from build123d import *

# Parameters (mm, degrees)
SKETCH2_R           = 12.5
SKETCH2_R_2         = 10
BOSS_EXTRUDE3_DEPTH = 90
SKETCH3_R           = 12.5
BOSS_EXTRUDE4_DEPTH = 30
BOSS_EXTRUDE5_DEPTH = 75


with BuildPart() as part:
    # Sketch2 → Boss-Extrude3 (new body)
    with BuildSketch(Plane(origin=(0, 0, 0), x_dir=(1, 0, 0), z_dir=(0, 1, 0))):
        with Locations(Location((0, 0, 0), (0, 0, 90))):
            Circle(SKETCH2_R)
        with Locations(Location((0, 0, 0), (0, 0, 90))):
            Circle(SKETCH2_R_2, mode=Mode.SUBTRACT)
    extrude(amount=BOSS_EXTRUDE3_DEPTH)

    # Sketch3 → Boss-Extrude4 (add)
    with BuildSketch(Plane(origin=(0, 90, 0), x_dir=(1, 0, 0), z_dir=(0, 1, 0))):
        with Locations(Location((0, 0, 0), (0, 0, 90))):
            Circle(SKETCH3_R)
    extrude(amount=BOSS_EXTRUDE4_DEPTH)

    # Sketch5 → Boss-Extrude5 (add, symmetric)
    with BuildSketch(Plane.XY):
        Polygon((-1, 90), (1, 90), (1, 120), (0, 165), (-1, 120), align=None)
    extrude(amount=BOSS_EXTRUDE5_DEPTH, both=True)


solid = part.part
The model under review builds one solid part; all positions refer to its coordinate system, in mm. A direction names the side the tool comes from. Round coordinates to 2 decimals unless told otherwise and drop trailing zeros. Write each loop counter-clockwise with the first axis right and the second up, starting at its lowest first coordinate (ties: lowest second). Pieces come first, ordered by that corner, then holes. Notation, with made-up numbers: M 86.5,-34.5 L 104.5,-34.5 A12 ccw 104.5,-17.5 Z; hole C 39,-1 d10. An arc over 180 degrees is marked long. Answer as CSV lines item,"result". Start each with the question number.
Q1. Consider section B-B, the plane z = 0. Give the boundary of the cut face in (x, y), then the cut area to 4 significant figures.
Q2. The part is to be moulded in two halves that separate along X. For faces 5 (the face through (1, 105, -43)), 6 (the face through (9.76, 44.37, 2.17)), 7 (the face through (5, 120, 0)), say which applies: +X half, -X half, draft (parallel to the pull), parting line (faces both ways), or undercut.
Q3. Consider section A-A, the plane y = 19. Give the boundary of the cut face in (x, z), then the cut area to 3 significant figures.
Q4. Wall thickness on line 1 along X through (y, z) = (29.5, 0); line 2 along Z through (x, y) = (6.75, 40); line 3 along Z through (x, y) = (-5.75, 21): over which ranges is each line inside the solid? List them lowest first.
Q5. Consider section C-C, the plane x = 5. Give the boundary of the cut face in (y, z).
Q6. Clearance check with flat-ended pins moving along their axes: P1, Ø9, axis at y = 111.5, z = 52, coming from the +X side; P2, Ø1, axis at x = -9, y = 94.5, coming from the -Z side; P3, Ø0.6, axis at x = 0, z = 36.5, coming from the -Y side. State where each tip first meets the part, or that it passes through.
Q7. Tool access review of faces 1 (the face through (1, 105, 44)), 2 (the face through (-1, 105, -43)), 3 (the face through (0, 90, 0)), 4 (the face through (-1, 105, 44)): name each direction out of +Z, -Z, +X, -X, +Y, -Y from which nothing blocks a thin tool from reaching the whole face with its end or side.
Q8. Consider section D-D, the plane z = 45. Give the boundary of the cut face in (x, y), then the cut area to 3 significant figures.
Result set:
1,outline,"M -12.5,0 L -10,0 L -10,90 L 10,90 L 10,0 L 12.5,0 L 12.5,120 L 1,120 L 0,165 L -1,120 L -12.5,120 Z"
1,area,"1,245 mm²"
2,face 5,"+X half"
2,face 6,"undercut"
2,face 7,"draft"
3,outline,"C 0,0 d25; hole C 0,0 d20"
3,area,"177 mm²"
4,line 1,"x = -12.5 to -10, 10 to 12.5"
4,line 2,"z = -10.52 to -7.38, 7.38 to 10.52"
4,line 3,"z = -11.1 to -8.18, 8.18 to 11.1"
5,outline,"M 0,-11.46 L 120,-11.46 L 120,11.46 L 0,11.46 L 0,8.66 L 90,8.66 L 90,-8.66 L 0,-8.66 Z"
6,P1,"stops at x = 1"
6,P2,"stops at z = -9.17"
6,P3,"stops at y = 90"
7,face 1,"+Z, +X, +Y, -Y"
7,face 2,"-Z, -X, +Y, -Y"
7,face 3,"-Y"
7,face 4,"+Z, -X, +Y, -Y"
8,outline,"M -1,90 L 1,90 L 1,120 L 0,165 L -1,120 Z"
8,area,"105 mm²"
